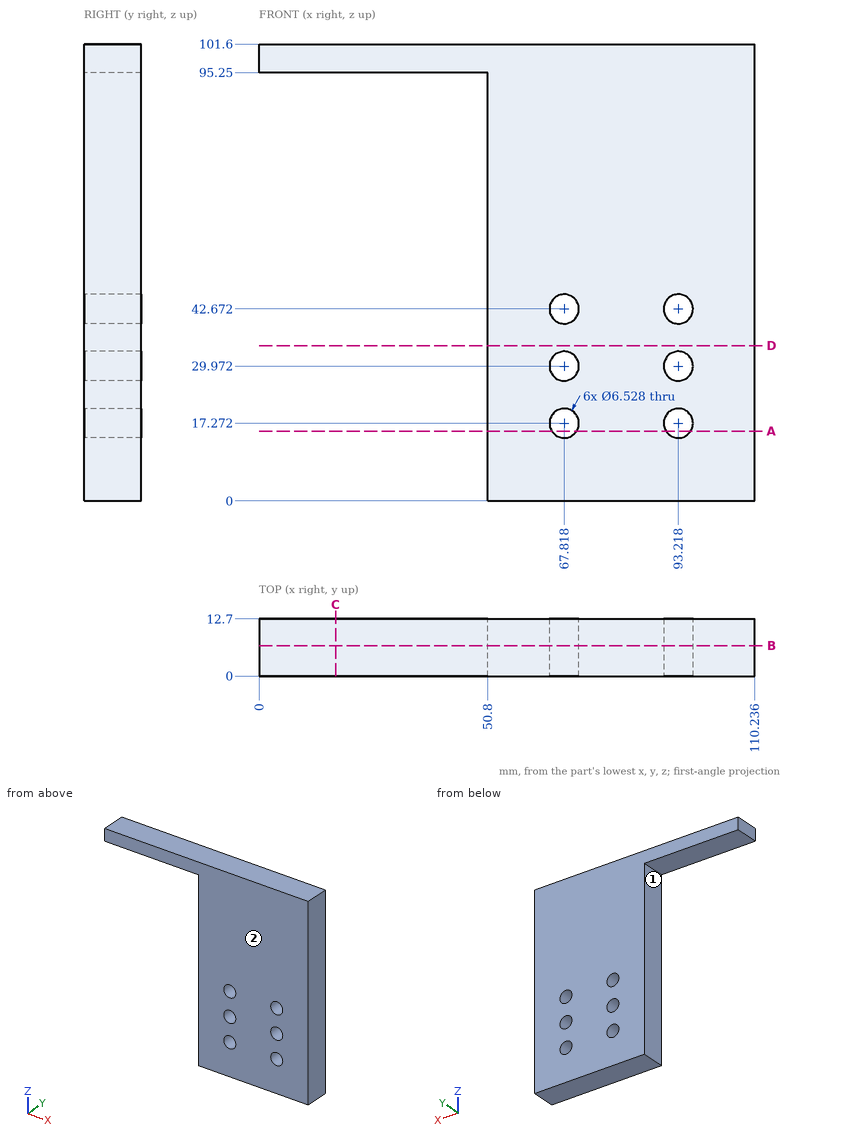
Print and shaded views of the part. All mm, measured from the part's lowest x, y and z. A direction names the side the tool comes from. Coordinates: 2 decimals unless noted, no trailing zeros. Order: outer loops, then holes, each group sorted by start corner. A loop starts at its lowest first (then second) coordinate and runs counter-clockwise, first axis right, second up. Notation, with made-up numbers: (-8.5, 87.5) - (-0.5, 87.5) arc R20 ccw to (-0.5, 94.5) - close; hole circle Ø1 at (-10.5, 52.25). An arc over 180 degrees is marked (long way). Return JSON: item names as keys, results as strings. Group by question number.
Item 1: Cut at A-A (z = 15.5). List the corners of the cut face in (x, y).
Item 2: Cut at B-B (y = 6.75). List the corners of the cut face in (x, z).
Item 3: Pin check, flat tips, straight feed: pin 1 (5 mm diameter, centred on x = 93.218, z = 17.272, fed in from +Y); pin 2 (2 mm diameter, centred on y = 9, z = 66.5, fed in from -X); pin 3 (6.5 mm diameter, centred on x = 23, y = 8.5, fed in from -Z). Stop position of each tip, or through.
Item 4: Cut at C-C (x = 17). List the corners of the cut face in (y, z).
Item 5: Which spindle directions (+Z, -Z, +X, -X, +Y, -Y) get a long thin tool onto all of the face, cutting with end or side? Do the marked faces 1 and 2. Say none if no direction does.
Item 6: Cut at D-D (z = 34.5). List the corners of the cut face in (x, y).
Item 7: Drill centre lines: probe 1 along X at (y, z) = (8, 17.5); probe 2 along X at (y, z) = (10.5, 29); probe 3 along X at (y, z) = (11.5, 37). Where is each one in solid material? Low to high. Write a range as from..to.
Check values:
{
 "1": {"outline": "(50.8, 0) - (65.08, 0) - (65.08, 12.7) - (50.8, 12.7) - close; (70.56, 0) - (90.48, 0) - (90.48, 12.7) - (70.56, 12.7) - close; (95.96, 0) - (110.24, 0) - (110.24, 12.7) - (95.96, 12.7) - close"},
 "2": {"outline": "(0, 95.25) - (50.8, 95.25) - (50.8, 0) - (110.24, 0) - (110.24, 101.6) - (0, 101.6) - close; hole circle Ø6.53 at (67.82, 17.27); hole circle Ø6.53 at (67.82, 29.97); hole circle Ø6.53 at (67.82, 42.67); hole circle Ø6.53 at (93.22, 17.27); hole circle Ø6.53 at (93.22, 29.97); hole circle Ø6.53 at (93.22, 42.67)"},
 "3": {"pin 1": "passes through", "pin 2": "stops at x = 50.8", "pin 3": "stops at z = 95.25"},
 "4": {"outline": "(0, 95.25) - (12.7, 95.25) - (12.7, 101.6) - (0, 101.6) - close"},
 "5": {"face 1": "-Z, -X, +Y, -Y", "face 2": "+Z, -Z, +X, -X, -Y"},
 "6": {"outline": "(50.8, 0) - (110.24, 0) - (110.24, 12.7) - (50.8, 12.7) - close"},
 "7": {"probe 1": "x = 50.8..64.56, 71.07..89.96, 96.47..110.24", "probe 2": "x = 50.8..64.7, 70.93..90.1, 96.33..110.24", "probe 3": "x = 50.8..110.24"}
}
